Part print with two shaded views. Sizes in mm from the minimum x, y, z corner. Round coordinates to 2 decimals unless told otherwise and drop trailing zeros. Order: outer loops, then holes, each group sorted by start corner. A loop starts at its lowest first (then second) coordinate and runs counter-clockwise, first axis right, second up. Notation, with made-up numbers: (3.25, -4.75) - (53.25, -4.75) arc R19 ccw to (53.25, 12.25) - close; hole circle Ø1 at (12, -6.5). An arc over 180 degrees is marked (long way). Answer as CSV lines item,"result". Start each with the question number.
1. Wall check: line 1 along X through (y, z) = (4.25, 92.5); line 2 along Z through (x, y) = (70, 4); line 3 along Y through (x, z) = (117.5, 90). Give the ranges that are in metal, low to high. Write a range as [from, to].
2. Band-saw the part on A-A on z = 92.5. List the corners of the cut face in (x, y), then the cut area to 3 significant figures.
3. Pin check, flat tips, straight feed: pin 1 Ø1 at (y, z) = (6.5, 75.5) entering from +X; pin 2 Ø8 at (x, z) = (64.85, 92.5) entering from +Y; pin 3 Ø3 at (y, z) = (4.5, 132.5) entering from -X. Stop position of each tip, or through.
4. Band-saw the part on B-B on x = 92.5. List the corners of the cut face in (y, z), then the cut area to 3 significant figures.
5. Band-saw the part on C-C on y = 8.25. State how many separate pieces and enclosed holes the cut face has, then the cut area to 3 significant figures.
6. Band-saw the part on D-D on z = 144. List the corners of the cut face in (x, y), then the cut area to 3 significant figures.
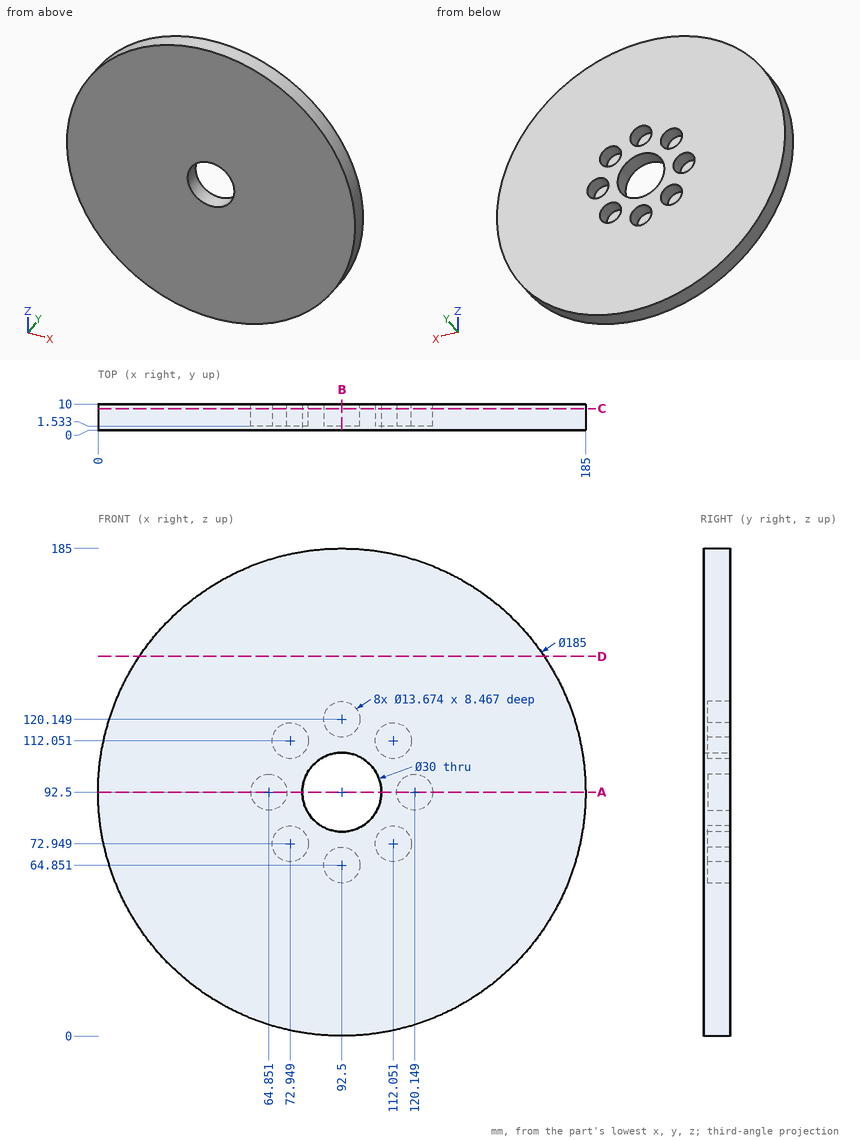
Reply:
1,line 1,"x = [0, 58.01], [71.69, 77.5], [107.5, 113.31], [126.99, 185]"
1,line 2,"z = [2.78, 66.78], [79.12, 88], [97, 105.88], [118.22, 182.22]"
1,line 3,"y = [0, 1.53]"
2,outline,"(0, 0) - (77.5, 0) - (77.5, 10) - (71.69, 10) - (71.69, 1.53) - (58.01, 1.53) - (58.01, 10) - (0, 10) - close; (107.5, 0) - (185, 0) - (185, 10) - (126.99, 10) - (126.99, 1.53) - (113.31, 1.53) - (113.31, 10) - (107.5, 10) - close"
2,area,"1,320 mm2"
3,pin 1,"stops at x = 183.52"
3,pin 2,"stops at y = 1.53"
3,pin 3,"stops at x = 8.39"
4,outline,"(0, 0) - (10, 0) - (10, 58.01) - (1.53, 58.01) - (1.53, 71.69) - (10, 71.69) - (10, 77.5) - (0, 77.5) - close; (0, 107.5) - (10, 107.5) - (10, 113.31) - (1.53, 113.31) - (1.53, 126.99) - (10, 126.99) - (10, 185) - (0, 185) - close"
4,area,"1,320 mm2"
5,separate pieces,"1"
5,enclosed holes,"9"
5,area,"25,000 mm2"
6,outline,"(15.66, 0) - (169.34, 0) - (169.34, 10) - (15.66, 10) - close"
6,area,"1,540 mm2"
